from build123d import *

# Parameters (mm, degrees)
BOSS_EXTRUDE1_DEPTH = 12
SKETCH4_W           = 57.71930009
SKETCH4_H           = 24
SKETCH4_R           = 4
BOSS_EXTRUDE2_DEPTH = 12
SKETCH4_3_R         = 8
SKETCH4_3_R_2       = 4
CUT_EXTRUDE1_DEPTH  = 5.15
FILLET1_R           = 12
SKETCH5_R           = 1.7
CUT_EXTRUDE2_DEPTH  = 113.615583531
CUT_EXTRUDE3_START  = -5
SKETCH5_3_R         = 3
CUT_EXTRUDE3_DEPTH  = 108.615583567


with BuildPart() as part:
    # Sketch3 → Boss-Extrude1 (new body)
    with BuildSketch(Plane(origin=(0, 0, 0), x_dir=(1, 0, 0), z_dir=(0, 1, 0))):
        with BuildLine():
            ThreePointArc((21.931712199, 12), (-25, 0), (21.931712199, -12))
            Line((21.931712199, -12), (61, -12))
            Line((61, -12), (61, 12))
            Line((61, 12), (21.931712199, 12))
        make_face()
        Polygon((-18.45, 10.652112467), (0, 21.304224933), (18.45, 10.652112467), (18.45, -10.652112467), (0, -21.304224933), (-18.45, -10.652112467), align=None, mode=Mode.SUBTRACT)
    extrude(amount=BOSS_EXTRUDE1_DEPTH)

    # Sketch4 → Boss-Extrude2 (add)
    with BuildSketch(Plane(origin=(30.5, -30.5, 0), x_dir=(0.7071067811865462, 0.7071067811865489, 0), z_dir=(0.7071067811865489, -0.7071067811865462, 0))):
        with Locations((71.993163697, 0)):
            Rectangle(SKETCH4_W, SKETCH4_H)
        with Locations((84.852813742, 0)):
            Circle(SKETCH4_R, mode=Mode.SUBTRACT)
    extrude(amount=-BOSS_EXTRUDE2_DEPTH)

    # Sketch4<3> → Cut-Extrude1 (cut)
    with BuildSketch(Plane(origin=(30.5, -30.5, 0), x_dir=(0.7071067811865462, 0.7071067811865489, 0), z_dir=(0.7071067811865489, -0.7071067811865462, 0))):
        with Locations((84.852813742, 0)):
            Circle(SKETCH4_3_R)
        with Locations((84.852813742, 0)):
            Circle(SKETCH4_3_R_2, mode=Mode.SUBTRACT)
    extrude(amount=-CUT_EXTRUDE1_DEPTH, mode=Mode.SUBTRACT)

    # Fillet1
    fillet1_edges = [part.edges().sort_by_distance(p)[0] for p in [
        (97.571067812, 45.056349186, -12),
        (97.571067812, 45.056349186, 12),
    ]]
    fillet(fillet1_edges, radius=FILLET1_R - 0.0001)  # a hair under: the kernel refuses the full size

    # Sketch5 → Cut-Extrude2 (cut, through all)
    with BuildSketch(Plane(origin=(9.225, 0, -15.9781687), x_dir=(0.8660254037844388, 0, 0.4999999999999997), z_dir=(-0.49999999999999983, 0, 0.8660254037844389))):
        with Locations((0, 6)):
            Circle(SKETCH5_R)
    cut_extrude2 = extrude(amount=-CUT_EXTRUDE2_DEPTH, mode=Mode.SUBTRACT)

    # Sketch5<3> → Cut-Extrude3 (cut, through all)
    with BuildSketch(Plane(origin=(9.225, 0, -15.9781687), x_dir=(0.8660254037844388, 0, 0.4999999999999997), z_dir=(-0.49999999999999983, 0, 0.8660254037844389)).offset(CUT_EXTRUDE3_START)):
        with Locations((0, 6)):
            Circle(SKETCH5_3_R)
    cut_extrude3 = extrude(amount=-CUT_EXTRUDE3_DEPTH, mode=Mode.SUBTRACT)

    # Mirror1: Cut-Extrude2, Cut-Extrude3 across plane
    add(cut_extrude2.mirror(Plane(origin=(0, 0, 0), x_dir=(0.866025403784439, 0, 0.4999999999999995), z_dir=(-0.49999999999999994, 0, 0.8660254037844388))), mode=Mode.SUBTRACT)
    add(cut_extrude3.mirror(Plane(origin=(0, 0, 0), x_dir=(0.866025403784439, 0, 0.4999999999999995), z_dir=(-0.49999999999999994, 0, 0.8660254037844388))), mode=Mode.SUBTRACT)


solid = part.part
Model file for the job. Use its own axes, mm. A direction names the side the tool comes from. Give positions to 0.01 mm unless a question says otherwise; leave off trailing zeros. Loops run counter-clockwise (first coordinate to the right, second up) from the corner with the lowest first, then second, coordinate; pieces in that order, holes last. Notation, with made-up numbers: (-11.75, 64) -> (22.25, 64) arc R23 ccw to (22.25, 87) -> close; hole circle Ø10 at (78.25, 24.25). An arc over 180 degrees is marked (long way). Use a Markdown table: item, result. Add a question column.
(1) Mould opens along Z. For faces 1 (the flat face through (74.42, 30.39, 0.17)), 2 (the cylindrical face through (94.96, 42.56, -8.58)), 3 (the flat face through (-11.76, 4.04, 20.29)), 4 (the cylindrical face through (95.09, 42.7, 8.39)) say: +Z half, -Z half, draft (parallel to the pull), parting line (faces both ways), or undercut.
(2) Slice it at C-C on z = -17.5. Give the number of separate pieces and of enclosed holes in the cut face, and give its area (3 significant figures).
(3) Slice it at D-D on z = 13.5. List the corners of the cut face in (x, y).
(4) Drop flat-ended pins along their axis: pin 1 Ø12 at (x, z) = (77.5, 8) entering from -Y; pin 2 Ø12 at (x, y) = (-10, 19) entering from -Z; pin 3 Ø4 at (y, z) = (12.5, 6.5) entering from +X; pin 4 Ø13 at (y, z) = (6, -0.5) entering from -X. Give the stop position or say it passes through.
(5) Tool access for faces 5 (the flat face through (89.293, 35.577, -3.444)), 6 (the flat face through (60, 14, -12)), 7 (the flat face through (60.1, 15.8, 12)), 8 (the flat face through (-18.45, 6, 0)), 9 (the flat face through (24, 12, 0)): list every direction of +Z, -Z, +X, -X, +Y, -Y with a clear straight run to the whole face (end or side of a thin tool).
(6) Slice it at A-A on z = 5.5. List the corners of the cut face in (x, y).
(7) Wall check: line 1 along Z through (x, y) = (80, 34); line 2 along X through (y, z) = (2.5, 19); line 3 along X through (y, z) = (2, -16.5). Give the ranges that are in metal, low to high.
(8) Slice it at B-B on x = 53. List the corners of the cut face in (y, z).
Filled sheet:
| question | item | result |
|---|---|---|
| 1 | face 1 | draft |
| 1 | face 2 | -Z half |
| 1 | face 3 | undercut |
| 1 | face 4 | +Z half |
| 2 | separate pieces | 2 |
| 2 | enclosed holes | 1 |
| 2 | area | 260 mm2 |
| 3 | outline | (-21.04, 0) -> (-13.52, 0) -> (-13.52, 12) -> (-21.04, 12) -> close; (13.52, 0) -> (21.04, 0) -> (21.04, 12) -> (13.52, 12) -> close |
| 4 | pin 1 | y = 10.5 |
| 4 | pin 2 | through |
| 4 | pin 3 | x = 75.5 |
| 4 | pin 4 | x = -25 |
| 5 | face 5 | none |
| 5 | face 6 | -Z, +X, +Y, -Y |
| 5 | face 7 | +Z, +X, +Y, -Y |
| 5 | face 8 | +Y, -Y |
| 5 | face 9 | +Z, -Z, -X, +Y |
| 6 | outline | (-24.39, 0) -> (-18.45, 0) -> (-18.45, 12) -> (-24.39, 12) -> close; (18.45, 0) -> (61, 0) -> (86.39, 25.39) -> (82.75, 29.03) -> (90.97, 37.25) -> (94.61, 33.61) -> (100.87, 39.87) -> (92.38, 48.36) -> (56.03, 12) -> (18.45, 12) -> close |
| 7 | line 1 | -12 to 12 |
| 7 | line 2 | -16.25 to -3.99, 3.99 to 16.25 |
| 7 | line 3 | -18.78 to -8.32, 8.32 to 18.78 |
| 8 | outline | (0, -12) -> (12, -12) -> (12, 12) -> (0, 12) -> close |
